Geometry: see drawing. Coordinates: mm, zero at the bounding-box minimum. A direction names the side the tool comes from. Round coordinates to 2 decimals unless told otherwise and drop trailing zeros. Loops run counter-clockwise (first coordinate to the right, second up) from the corner with the lowest first, then second, coordinate; pieces in that order, holes last. Notation, with made-up numbers: (23, -32) - (35, -32) arc R29 cw to (35, -10) - close; hole circle Ø5 at (27, -11). An arc over 180 degrees is marked (long way). One line per question, with ' | ' between items. Start each with the question number.
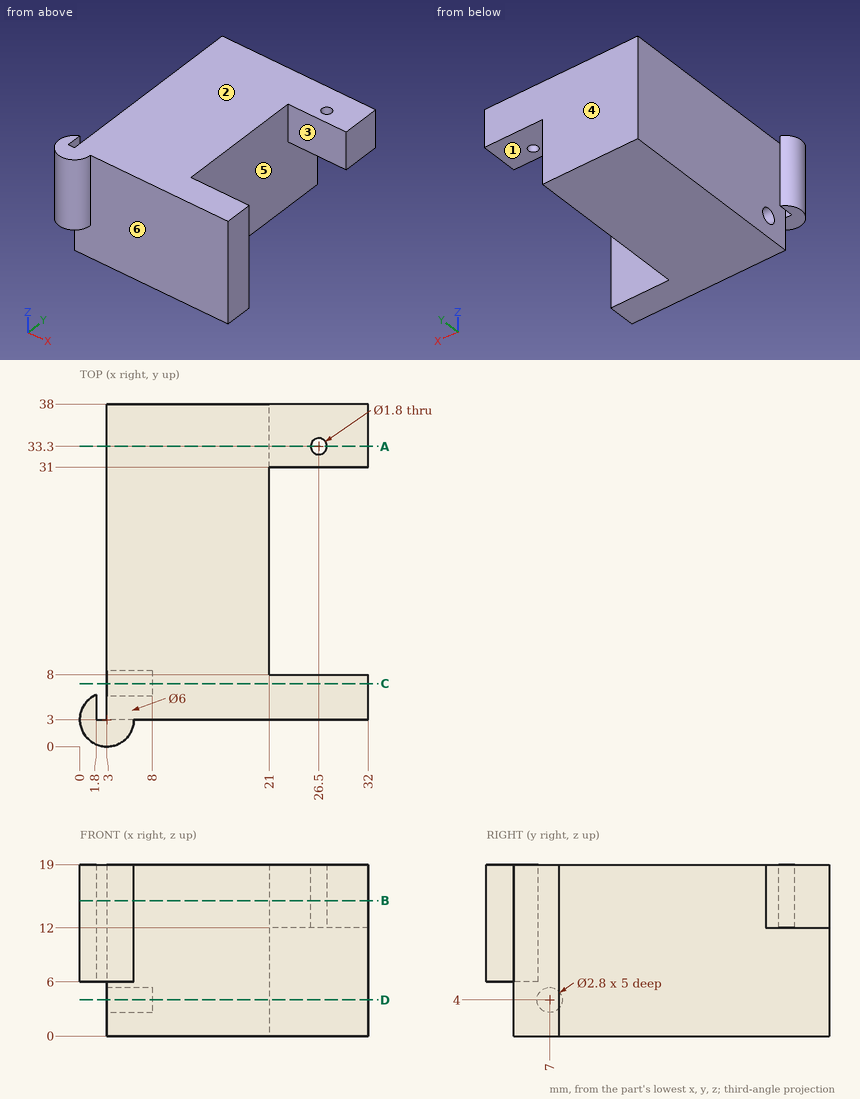
(1) Section B-B, the plane z = 15. Output: boundary loops of the cut face in (x, y).
(2) Section C-C, the plane y = 7. Output: boundary loops of the cut face in (x, z).
(3) Section D-D, the plane z = 4. Output: boundary loops of the cut face in (x, y), plus the area to 3 significant figures.
(4) Reachability of the marked faces 1, 2 and 3 from +Z, -Z, +X, -X, +Y, -Y: full face, straight path, thin tool, end or side. Return the list, or none.
(5) Section A-A, the plane y = 33.3. Output: boundary loops of the cut face in (x, z), plus the area to 3 significant figures.
(6) Line query: line 1 along X through (y, z) = (33.3, 17.5); line 2 along X through (y, z) = (15.5, 4); line 3 along Y through (x, z) = (8, 12). Output: solid intervals per line, ascending. Write a range as from..to.
(7) Pull-direction query (Y, two-part tool) for the marked faces 4, 5 and 6; classes: released by +Y, released by -Y, zero draft, split by the parting line, or undercut.
(8) Pin query (flat end, axial travel): P1, Ø3, axis at y = 6.5, z = 4, coming from the -X side; P2, Ø2, axis at y = 16, z = 13, coming from the +X side; P3, Ø1.7, axis at x = 2.5, y = 1.5, coming from the -Z side. Return the tip coordinate at first contact, or that it passes through.
Derived:
1) outline: (1.8, 3) - (1.8, 5.75) arc R3 ccw (long way) to (6, 3) - (32, 3) - (32, 8) - (21, 8) - (21, 31) - (32, 31) - (32, 38) - (3, 38) - (3, 3) - close; hole circle Ø1.8 at (26.5, 33.3)
2) outline: (3, 0) - (32, 0) - (32, 19) - (3, 19) - (3, 5.4) - (8, 5.4) - (8, 2.6) - (3, 2.6) - close
3) outline: (3, 3) - (32, 3) - (32, 8) - (21, 8) - (21, 38) - (3, 38) - (3, 8.4) - (8, 8.4) - (8, 5.6) - (3, 5.6) - close | area: 671 mm²
4) face 1: -Z, +X, +Y | face 2: +Z, +X, -X, +Y, -Y | face 3: +Z, -Z, +X
5) outline: (3, 0) - (21, 0) - (21, 12) - (25.6, 12) - (25.6, 19) - (3, 19) - close; (27.4, 12) - (32, 12) - (32, 19) - (27.4, 19) - close | area: 406 mm²
6) line 1: x = 3..25.6, 27.4..32 | line 2: x = 3..21 | line 3: y = 3..38
7) face 4: released by +Y | face 5: undercut | face 6: released by -Y
8) P1: stops at x = 3 | P2: stops at x = 21 | P3: stops at z = 6
